Geometry: final body of the model. Coordinates: model frame, mm. Face numbers are marked on the shaded views. A direction names the side the tool comes from. Coordinates: 2 decimals unless noted, no trailing zeros. Order: outer loops, then holes, each group sorted by start corner. A loop starts at its lowest first (then second) coordinate and runs counter-clockwise, first axis right, second up. Notation, with made-up numbers: M -16,52.25 L 40,52.25 A21 cw 40,66.25 Z; hole C -30.75,-12 d3. An arc over 180 degrees is marked long. One line per question, with ' | ' between items.
from build123d import *

# Parameters (mm, degrees)
SKETCH_1_W          = 10
SKETCH_1_H          = 10
SKETCH_1_W_2        = 7
SKETCH_1_H_2        = 7
EXTRUDE_1_DEPTH     = 60
SKETCH_2_R          = 1.6
CUT_EXTRUDE_1_DEPTH = 62.032778079
SKETCH_3_R          = 2.15
CUT_EXTRUDE_2_DEPTH = 62.032778079


with BuildPart() as part:
    # ｽｹｯﾁ1 → 押し出し-薄板1 (new body)
    with BuildSketch(Plane(origin=(0, 0, 0), x_dir=(1, 0, 0), z_dir=(0, 1, 0))):
        Rectangle(SKETCH_1_W, SKETCH_1_H)
        Rectangle(SKETCH_1_W_2, SKETCH_1_H_2, mode=Mode.SUBTRACT)
    extrude(amount=EXTRUDE_1_DEPTH)

    # ｽｹｯﾁ2 → ｶｯﾄ - 押し出し1 (cut, through all)
    with BuildSketch(Plane.XY.offset(5)):
        with Locations((0, 25)):
            Circle(SKETCH_2_R)
        with Locations((0, 5)):
            Circle(SKETCH_2_R)
    extrude(amount=-CUT_EXTRUDE_1_DEPTH, mode=Mode.SUBTRACT)

    # ｽｹｯﾁ3 → ｶｯﾄ - 押し出し2 (cut, through all)
    with BuildSketch(Plane(origin=(5, 0, 0), x_dir=(0, 0, -1), z_dir=(1, 0, 0))):
        with Locations((0, 55)):
            Circle(SKETCH_3_R)
    extrude(amount=-CUT_EXTRUDE_2_DEPTH, mode=Mode.SUBTRACT)


solid = part.part
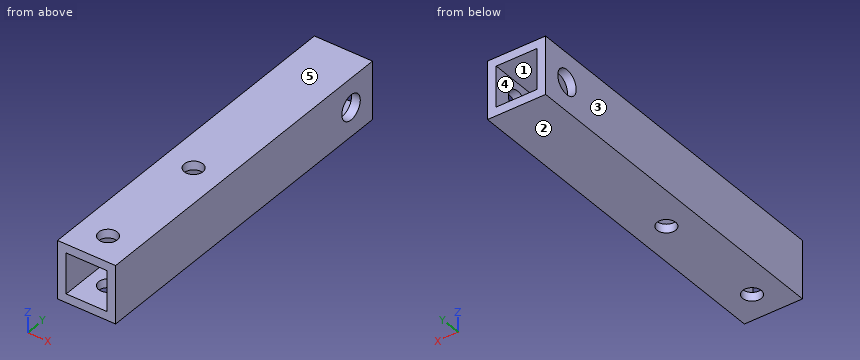
1. Section B-B, the plane y = 5. Output: boundary loops of the cut face in (x, z), and give its area (3 significant figures).
Response values:
outline: M -5,-5 L -1.6,-5 L -1.6,-3.5 L -3.5,-3.5 L -3.5,3.5 L -1.6,3.5 L -1.6,5 L -5,5 Z; M 1.6,-5 L 5,-5 L 5,5 L 1.6,5 L 1.6,3.5 L 3.5,3.5 L 3.5,-3.5 L 1.6,-3.5 Z | area: 41.4 mm^2
2. Section A-A, the plane x = 0. Output: boundary loops of the cut face in (y, z), and give its area (3 significant figures).
Response values:
outline: M 0,-5 L 3.4,-5 L 3.4,-3.5 L 0,-3.5 Z; M 0,3.5 L 3.4,3.5 L 3.4,5 L 0,5 Z; M 6.6,-5 L 23.4,-5 L 23.4,-3.5 L 6.6,-3.5 Z; M 6.6,3.5 L 23.4,3.5 L 23.4,5 L 6.6,5 Z; M 26.6,-5 L 60,-5 L 60,-3.5 L 26.6,-3.5 Z; M 26.6,3.5 L 60,3.5 L 60,5 L 26.6,5 Z | area: 161 mm^2
3. Access query for the marked faces 1 and 2. Directions: +Z, -Z, +X, -X, +Y, -Y. A direction counts if a zero-diameter tool reaches every point of the face in a straight line with its end or side. Return the directions, or none.
Response values:
face 1: +Y, -Y | face 2: -Z, +X, -X, +Y, -Y
4. Section D-D, the plane y = 20.5. Output: boundary loops of the cut face in (x, z).
Response values:
outline: M -5,-5 L 5,-5 L 5,5 L -5,5 Z; hole M -3.5,-3.5 L 3.5,-3.5 L 3.5,3.5 L -3.5,3.5 Z
5. Section C-C, the plane z = -2.75. Output: boundary loops of the cut face in (x, y).
Response values:
outline: M -5,0 L -3.5,0 L -3.5,60 L -5,60 Z; M 3.5,0 L 5,0 L 5,60 L 3.5,60 Z
6. Pin query (flat end, axial travel): P1, Ø5, axis at x = 0, y = 25, coming from the +Z side; P2, Ø2.5, axis at y = 55, z = 0, coming from the -X side. Return the tip coordinate at first contact, or that it passes through.
Response values:
P1: stops at z = 5 | P2: passes through
7. Material intervals for line 1 (Y direction, x = 0, z = -4.6); line 2 (Z direction, x = 0.5, y = 36.5), sorted ascending. Write a range as [from, to].
Response values:
line 1: y = [0, 3.4], [6.6, 23.4], [26.6, 60] | line 2: z = [-5, -3.5], [3.5, 5]
8. Draft query along X for the marked faces 3, 4 and 5. Return one class per face: pulls with the +X half, pulls with the -X half, needs draft (parallel to the pull), parting line crosses it, or undercut.
Response values:
face 3: pulls with the -X half | face 4: undercut | face 5: needs draft
